Autodesk Inventor part; units mm, degrees
ref_plane "YZ Plane" through (0, 0, 0) normal (1, 0, 0) x (0, 1, 0)
ref_plane "XZ Plane" through (0, 0, 0) normal (0, 1, 0) x (-1, 0, 0)
ref_plane "XY Plane" through (0, 0, 0) normal (0, 0, 1) x (1, 0, 0)
sketch "Sketch1" plane through (0, 0, 0) normal (1, 0, 0) x (0, 1, 0)
  line L0 (228.6, 381) -> (-228.6, 381)
  line L1 (-228.6, 381) -> (-228.6, -381)
  line L2 (-228.6, -381) -> (228.6, -381)
  line L3 (228.6, -381) -> (228.6, 381)
  point P0 (0, 0)
  point P1 (228.6, 0)
  point P2 (0, -381)
  dimension "d0" = 762
  dimension "d1" = 457.2
extrude "Extrusion1" add sketch "Sketch1" along normal blind 50.8
sketch "Sketch2" plane through (50.8, 0, 0) normal (1, 0, 0) x (0, 0, -1)
  line L0 (381, 228.6) -> (-381, 228.6)
  line L1 (-381, 228.6) -> (-381, -228.6)
  line L2 (-381, -228.6) -> (381, -228.6)
  line L3 (381, -228.6) -> (381, 228.6)
  line L4 (-355.6, 203.2) -> (355.6, 203.2)
  line L5 (355.6, 203.2) -> (355.6, -203.2)
  line L6 (355.6, -203.2) -> (-355.6, -203.2)
  line L7 (-355.6, -203.2) -> (-355.6, 203.2)
  point P0 (0, 0)
  dimension "d4" = 25.4
extrude "Extrusion2" cut sketch "Sketch2" against normal blind 2.54 contours L4 L5 L6 L7
properties part number "Television"
CAD build for the part. Positions are in the model's coordinates, mm. Round coordinates to 2 decimals unless told otherwise and drop trailing zeros. Loops run counter-clockwise (first coordinate to the right, second up) from the corner with the lowest first, then second, coordinate; pieces in that order, holes last. Notation, with made-up numbers: (25.5, 33) - (60.5, 33) arc R15 cw to (60.5, 57) - close; hole circle Ø8 at (48, 27). An arc over 180 degrees is marked (long way). Return JSON: item names as keys, results as strings. Group by question number.
Q1. Band-saw the part on B-B on z = -8.5. Give the cut face in (x, y), plus the area to 3 significant figures.
Q2. Drill centre line: line 1 along X through (y, z) = (5, -21.5). Where is it in solid material? Low to high. Write a range as [from, to].
Q3. Two-plate mould, pull along Y, no slides. Class faces 1 (the face through (50.8, -204, 2)), 2 (the face through (25, -228.6, 5)), 3 (the face through (25, 228.6, -5)), 4 (the face through (48.26, 3, 5)): +Y half, -Y half, draft (parallel to the pull), parting line (faces both ways), or undercut.
Q4. Band-saw the part on A-A on y = 170.5. Give the cut face in (x, z).
Q5. Flat gauge pin, fed straight in: pin 1 Ø12 at (y, z) = (-93.5, -8) entering from +X. Where does the tip first touch, or does it go through?
Solutions:
{
 "1": {"outline": "(0, -228.6) - (50.8, -228.6) - (50.8, -203.2) - (48.26, -203.2) - (48.26, 203.2) - (50.8, 203.2) - (50.8, 228.6) - (0, 228.6) - close", "area": "22,200 mm^2"},
 "2": {"line 1": "x = [0, 48.26]"},
 "3": {"face 1": "draft", "face 2": "-Y half", "face 3": "+Y half", "face 4": "undercut"},
 "4": {"outline": "(0, -381) - (50.8, -381) - (50.8, -355.6) - (48.26, -355.6) - (48.26, 355.6) - (50.8, 355.6) - (50.8, 381) - (0, 381) - close"},
 "5": {"pin 1": "stops at x = 48.26"}
}
